from build123d import *

# Parameters (mm, degrees)
CROQUIS1_W              = 190
CROQUIS1_H              = 280
SALIENTE_EXTRUIR1_DEPTH = 105
CROQUIS2_W              = 73
CROQUIS2_H              = 75
CROQUIS2_W_2            = 53
CROQUIS2_H_2            = 61
SALIENTE_EXTRUIR2_DEPTH = 10
CROQUIS3_W              = 190
CROQUIS3_H              = 32
CORTAR_EXTRUIR1_DEPTH   = 5
CROQUIS4_W              = 190
CROQUIS4_H              = 61
CORTAR_EXTRUIR2_DEPTH   = 3
CORTAR_EXTRUIR3_DEPTH   = 53
SALIENTE_EXTRUIR3_DEPTH = 53
CORTAR_EXTRUIR4_DEPTH   = 2
CORTAR_EXTRUIR5_DEPTH   = 2
CROQUIS10_W             = 190
CROQUIS10_H             = 44
CORTAR_EXTRUIR6_DEPTH   = 3
CROQUIS11_W             = 190
CROQUIS11_H             = 37
CORTAR_EXTRUIR7_DEPTH   = 5


with BuildPart() as part:
    # Croquis1 → Saliente-Extruir1 (new body)
    with BuildSketch(Plane.XY):
        Rectangle(CROQUIS1_W, CROQUIS1_H)
    extrude(amount=SALIENTE_EXTRUIR1_DEPTH)

    # Croquis2 → Saliente-Extruir2 (add)
    with BuildSketch(Plane.XY.offset(105)):
        with Locations((0, -12.5)):
            Rectangle(CROQUIS2_W, CROQUIS2_H)
        with Locations((0, -12.5)):
            Rectangle(CROQUIS2_W_2, CROQUIS2_H_2, mode=Mode.SUBTRACT)
    extrude(amount=SALIENTE_EXTRUIR2_DEPTH)

    # Croquis3 → Cortar-Extruir1 (cut)
    with BuildSketch(Plane.XY.offset(105)):
        with Locations((0, 120)):
            Rectangle(CROQUIS3_W, CROQUIS3_H)
    extrude(amount=-CORTAR_EXTRUIR1_DEPTH, mode=Mode.SUBTRACT)

    # Croquis4 → Cortar-Extruir2 (cut)
    with BuildSketch(Plane.XY.offset(105)):
        with Locations((0, 73.5)):
            Rectangle(CROQUIS4_W, CROQUIS4_H)
    extrude(amount=-CORTAR_EXTRUIR2_DEPTH, mode=Mode.SUBTRACT)

    # Croquis6 → Cortar-Extruir3 (cut)
    with BuildSketch(Plane(origin=(-26.5, 0, 0), x_dir=(0, 0, -1), z_dir=(1, 0, 0))):
        with BuildLine():
            Line((-105, 18), (-101, 18))
            ThreePointArc((-101, 18), (-105, -12.5), (-101, -43))
            Line((-101, -43), (-105, -43))
            Line((-105, -43), (-107.940115758, -14.951898157))
            Line((-107.940115758, -14.951898157), (-105, 18))
        make_face()
    extrude(amount=CORTAR_EXTRUIR3_DEPTH, mode=Mode.SUBTRACT)

    # Croquis7 → Saliente-Extruir3 (add)
    with BuildSketch(Plane(origin=(-26.5, 0, 0), x_dir=(0, 0, -1), z_dir=(1, 0, 0))):
        with BuildLine():
            Line((-103.681451712, 5.111942251), (-135, 6.21315585))
            Line((-135, 6.21315585), (-135.421940476, -5.78684415))
            Line((-135.421940476, -5.78684415), (-104.965398794, -9.639204549))
            ThreePointArc((-104.965398794, -9.639204549), (-104.554477707, -2.24352023), (-103.681451712, 5.111942251))
        make_face()
    extrude(amount=SALIENTE_EXTRUIR3_DEPTH)

    # Croquis8 → Cortar-Extruir4 (cut)
    with BuildSketch(Plane(origin=(26.5, 0, 0), x_dir=(0, 0, -1), z_dir=(1, 0, 0))):
        with BuildLine():
            Line((-135, 6.21315585), (-103.681451712, 5.111942251))
            ThreePointArc((-103.681451712, 5.111942251), (-104.652420764, -2.234995218), (-104.965398794, -9.639204549))
            Line((-104.965398794, -9.639204549), (-135.421940476, -5.78684415))
            Line((-135.421940476, -5.78684415), (-135, 6.21315585))
        make_face()
    extrude(amount=-CORTAR_EXTRUIR4_DEPTH, mode=Mode.SUBTRACT)

    # Croquis9 → Cortar-Extruir5 (cut)
    with BuildSketch(Plane.ZY.offset(26.5)):
        with BuildLine():
            Line((103.681451712, 5.111942251), (135, 6.21315585))
            Line((135, 6.21315585), (135.421940476, -5.78684415))
            Line((135.421940476, -5.78684415), (104.965398794, -9.639204549))
            ThreePointArc((104.965398794, -9.639204549), (104.652420764, -2.234995218), (103.681451712, 5.111942251))
        make_face()
    extrude(amount=-CORTAR_EXTRUIR5_DEPTH, mode=Mode.SUBTRACT)

    # Croquis10 → Cortar-Extruir6 (cut)
    with BuildSketch(Plane.XY.offset(105)):
        with Locations((0, -76)):
            Rectangle(CROQUIS10_W, CROQUIS10_H)
    extrude(amount=-CORTAR_EXTRUIR6_DEPTH, mode=Mode.SUBTRACT)

    # Croquis11 → Cortar-Extruir7 (cut)
    with BuildSketch(Plane.XY.offset(105)):
        with Locations((0, -116.5)):
            Rectangle(CROQUIS11_W, CROQUIS11_H)
    extrude(amount=-CORTAR_EXTRUIR7_DEPTH, mode=Mode.SUBTRACT)


solid = part.part
Geometry: final body of the model. Coordinates: model frame, mm. A direction names the side the tool comes from. Give positions to 0.01 mm unless a question says otherwise; leave off trailing zeros. Write each loop counter-clockwise with the first axis right and the second up, starting at its lowest first coordinate (ties: lowest second). Pieces come first, ordered by that corner, then holes. Notation, with made-up numbers: (-2.75, 81) -> (1.25, 81) arc R15 ccw to (1.25, 92) -> close; hole circle Ø4 at (-13, 64). An arc over 180 degrees is marked (long way). Answer as a JSON object with one key per item and string values.
1. Access query for faces 5 (the flat face through (-1, 74, 102)), 6 (the flat face through (36.5, -13, 110)), 7 (the flat face through (24.5, -2, 119)). Directions: +Z, -Z, +X, -X, +Y, -Y. A direction counts if a zero-diameter tool reaches every point of the face in a straight line with its end or side. Return the directions, or none.
Ans:
{"face 5": "+Z, +X, -X", "face 6": "+Z, +X, +Y, -Y", "face 7": "+Z"}
2. Cut plane B-B on x = -61.5. Output: boundary loops of the cut face in (y, z).
Ans:
{"outline": "(-140, 0) -> (140, 0) -> (140, 105) -> (136, 105) -> (136, 100) -> (104, 100) -> (104, 102) -> (43, 102) -> (43, 105) -> (-54, 105) -> (-54, 102) -> (-98, 102) -> (-98, 100) -> (-135, 100) -> (-135, 105) -> (-140, 105) -> close"}
3. Contact query for flat-ended pins moving along their axis: pin 1 (12 mm diameter, centred on x = 63.5, y = -13.5, fed in from +Z); pin 2 (8 mm diameter, centred on y = -30, z = 110, fed in from +X); pin 3 (3 mm diameter, centred on y = 0.5, z = 107.5, fed in from -X). Output: stop coordinate, or through.
Ans:
{"pin 1": "stops at z = 105", "pin 2": "stops at x = 36.5", "pin 3": "stops at x = -36.5"}
4. Ray query, probe 1 along X at (y, z) = (0, 114.5); probe 2 along Z at (x, y) = (82.5, 78); probe 3 along X at (y, z) = (-6.5, 122). Return the intervals inside material, ascending. Write a range as from..to.
Ans:
{"probe 1": "x = -36.5..-26.5, -24.5..24.5, 26.5..36.5", "probe 2": "z = 0..102", "probe 3": "x = -24.5..24.5"}
5. Mould query, pull axis X, two halves, no side actions, for faces 1 (the flat face through (-24.5, -2, 120)), 2 (the flat face through (-1, 25, 110)), 3 (the flat face through (-0.343, -7.686, 120.407)), 4 (the flat face through (-36.5, -13, 110)). Classes: pulls with the +X half, pulls with the -X half, needs draft (parallel to the pull), parting line crosses it, or undercut.
Ans:
{"face 1": "undercut", "face 2": "needs draft", "face 3": "undercut", "face 4": "pulls with the -X half"}
6. Cut plane C-C on y = 11. Output: boundary loops of the cut face in (x, z).
Ans:
{"outline": "(-95, 0) -> (95, 0) -> (95, 105) -> (36.5, 105) -> (36.5, 115) -> (26.5, 115) -> (26.5, 102.64) -> (-26.5, 102.64) -> (-26.5, 115) -> (-36.5, 115) -> (-36.5, 105) -> (-95, 105) -> close"}
7. Cut plane D-D on x = 19.5. Output: boundary loops of the cut face in (y, z).
Ans:
{"outline": "(-140, 0) -> (140, 0) -> (140, 105) -> (136, 105) -> (136, 100) -> (104, 100) -> (104, 102) -> (43, 102) -> (43, 105) -> (25, 105) -> (25, 115) -> (18, 115) -> (18, 101) arc R118.28 ccw to (5.11, 103.68) -> (6.21, 135) -> (-5.79, 135.42) -> (-9.64, 104.97) arc R118.28 ccw to (-43, 101) -> (-43, 115) -> (-50, 115) -> (-50, 105) -> (-54, 105) -> (-54, 102) -> (-98, 102) -> (-98, 100) -> (-135, 100) -> (-135, 105) -> (-140, 105) -> close"}
8. Cut plane A-A on z = 111. Output: boundary loops of the cut face in (x, y), and give its area (3 significant figures).
Ans:
{"outline": "(-36.5, -50) -> (36.5, -50) -> (36.5, 25) -> (-36.5, 25) -> close; (-24.5, -8.88) -> (24.5, -8.88) -> (24.5, 5.37) -> (-24.5, 5.37) -> close; hole (-26.5, -43) -> (26.5, -43) -> (26.5, 18) -> (-26.5, 18) -> close", "area": "2,940 mm^2"}
